Here's how the part is built. I have some questions about the finished solid (model axes, mm). Coordinates: 2 decimals unless noted, no trailing zeros. Loops run counter-clockwise (first coordinate to the right, second up) from the corner with the lowest first, then second, coordinate; pieces in that order, holes last. Notation, with made-up numbers: (81.5, 53.25) -> (126.5, 53.25) arc R31 ccw to (126.5, 83.25) -> close; hole circle Ø4 at (61, 71.25). An arc over 180 degrees is marked (long way). Answer as a JSON object with one key per item and string values. Group by question number.
1) I want a section at B-B (z = 2.25). Count the separate pieces of the cut face and the enclosed holes in it, then the cut area to 3 significant figures.
2) I need wall thicknesses on probe 1 along Y at (x, z) = (217, 1.25); probe 2 along X at (y, z) = (39, 1.25); probe 3 along Y at (x, z) = (42.5, 4.7). Which ranges of each line are inside material? Lowest first, please. Write a range as [from, to].
3) I want a section at A-A (y = 19). Write out the boundary of the cut face in (x, z).
4) I'm going to push flat-ended pins straight in: pin 1 (0.8 mm diameter, centred on x = 124, z = 3, fed in from +Y); pin 2 (2.5 mm diameter, centred on x = 99, z = 4, fed in from -Y); pin 3 (0.9 mm diameter, centred on x = 207.5, z = 3, fed in from -Y). Where does each tip first touch, or does it pass through?
Autodesk Inventor part; units mm, degrees
ref_plane "YZ Plane" through (0, 0, 0) normal (1, 0, 0) x (0, 1, 0)
ref_plane "XZ Plane" through (0, 0, 0) normal (0, 1, 0) x (-1, 0, 0)
ref_plane "XY Plane" through (0, 0, 0) normal (0, 0, 1) x (1, 0, 0)
sketch "Эскиз1" plane through (0, 0, 0) normal (0, 0, 1) x (1, 0, 0)
  line L0 (220, 84) -> (220, 0)
  line L1 (220, 0) -> (0, 0)
  line L2 (0, 0) -> (0, 84)
  line L3 (6, 0) -> (0, 0)
  line L4 (0, 76) -> (6, 76)
  line L5 (6, 76) -> (6, 8)
  line L6 (6, 8) -> (0, 8)
  line L7 (0, 8) -> (0, 76)
  ellipse E0 centre (95, 84) end of major axis (170, 84) minor radius 28.3094 (20, 84) -> (170, 84) ccw
  line L8 (0, 84) -> (20, 84)
  line L9 (170, 84) -> (220, 84)
  line L10 (220, 76) -> (214, 76)
  line L11 (214, 76) -> (214, 8)
  line L12 (214, 8) -> (220, 8)
  line L13 (220, 8) -> (220, 76)
  line L14 (0, 68) -> (6, 68)
  line L15 (6, 68) -> (6, 52)
  line L16 (6, 52) -> (0, 52)
  line L17 (0, 52) -> (0, 68)
  line L18 (0, 32) -> (6, 32)
  line L19 (6, 32) -> (6, 16)
  line L20 (6, 16) -> (0, 16)
  line L21 (0, 16) -> (0, 32)
  line L22 (214, 68) -> (220, 68)
  line L23 (214, 52) -> (220, 52)
  line L24 (214, 32) -> (220, 32)
  line L25 (214, 16) -> (220, 16)
  line L26 (0, 84) -> (-6, 84)
  line L27 (-6, 84) -> (-6, 0)
  line L28 (-6, 0) -> (0, 0)
  line L29 (0, 0) -> (0, 84)
  line L30 (220, 84) -> (226, 84)
  line L31 (226, 84) -> (226, 0)
  line L32 (226, 0) -> (220, 0)
  line L33 (220, 0) -> (220, 84)
  point P0 (217, 8)
  point P1 (220, 8)
  point P2 (3, 76)
  point P3 (3, 0)
  point P4 (217, 76)
  point P5 (3, 68)
  point P6 (0, 16)
  point P7 (0, 52)
  point P8 (217, 68)
  point P9 (217, 32)
  point P10 (217, 16)
  point P11 (217, 52)
  point P12 (220, 32)
  point P13 (220, 52)
  point P14 (220, 68)
  dimension "d1" = 75
  dimension "d0" = 220
  dimension "d2" = 125
  dimension "d3" = 84
  dimension "d4" = 150
  dimension "d5" = 84
  dimension "d6" = 6
  dimension "d7" = 8
  dimension "d10" = 6
  dimension "d11" = 8
  dimension "d12" = 8
  dimension "d13" = 8
  dimension "d14" = 84
  dimension "d35" = 8
  dimension "d36" = 8
  dimension "d37" = 16
  dimension "d38" = 16
  dimension "d39" = 8
  dimension "d40" = 8
  dimension "d41" = 16
  dimension "d42" = 16
  dimension "d96" = 6
  dimension "d97" = 6
extrude "Выдавливание1" add sketch "Эскиз1" along normal blind 6 contours L30 L31 L32 L0 | L0 L10 L11 L12 L1 L2 L6 L5 L4 L8 E0 L9 | L0 L23 L11 L22 | L2 L28 L27 L26 | L0 L25 L11 L24 | L14 L5 L16 L2 | L18 L5 L20 L2
sketch "Эскиз2" plane through (0, 0, 6) normal (0, 0, 1) x (1, 0, 0)
  line L0 (0, 0) -> (220, 0)
  line L1 (6, 0) -> (48, 0)
  line L2 (48, 0) -> (48, 8)
  line L3 (48, 8) -> (6, 8)
  line L4 (6, 8) -> (6, 0)
  line L5 (48, 0) -> (40, 0)
  line L6 (40, 0) -> (40, 42)
  line L7 (40, 42) -> (48, 42)
  line L8 (48, 42) -> (48, 0)
  line L9 (48, 42) -> (6, 42)
  line L10 (6, 42) -> (6, 34)
  line L11 (6, 34) -> (48, 34)
  line L12 (48, 34) -> (48, 42)
  line L13 (6, 42) -> (14, 42)
  line L14 (14, 42) -> (14, 0)
  line L15 (14, 0) -> (6, 0)
  line L16 (6, 0) -> (6, 42)
  line L17 (6, 16) -> (6, 8)
  circle A0 centre (11.5, 36.5) radius 1.5
  circle A1 centre (42.5, 36.5) radius 1.5
  circle A2 centre (42.5, 5.5) radius 1.5
  circle A3 centre (11.5, 5.5) radius 1.5
  circle A4 centre (184, 19) radius 7
  circle A5 centre (177, 25.9159) radius 1.5
  circle A6 centre (191, 26.0852) radius 1.5
  circle A7 centre (191, 12) radius 1.5
  circle A8 centre (177, 12) radius 1.5
  line L18 (177, 42.7055) -> (177, 0) construction
  line L19 (173.1146, 12) -> (210.5161, 12) construction
  line L20 (0, 0) -> (220, 0)
  line L21 (174.3072, 25.8833) -> (201.7049, 26.2146) construction
  line L22 (191, 29.1476) -> (191, 5.5) construction
  line L23 (214, 8) -> (214, 16)
  circle A9 centre (27, 21) radius 12.5
  point P0 (27, 0)
  point P1 (6, 76)
  point P2 (14, 34)
  point P3 (14, 8)
  point P4 (40, 8)
  point P5 (40, 34)
  dimension "d15" = 42
  dimension "d16" = 42
  dimension "d17" = 8
  dimension "d18" = 8
  dimension "d19" = 8
  dimension "d20" = 8
  dimension "d21" = 3
  dimension "d22" = 3
  dimension "d23" = 3
  dimension "d24" = 3
  dimension "d25" = 5.5
  dimension "d26" = 5.5
  dimension "d27" = 5.5
  dimension "d28" = 5.5
  dimension "d29" = 5.5
  dimension "d30" = 5.5
  dimension "d31" = 5.5
  dimension "d32" = 5.5
  dimension "d78" = 14
  dimension "d80" = 3
  dimension "d81" = 3
  dimension "d82" = 3
  dimension "d83" = 3
  dimension "d91" = 30
  dimension "d93" = 21
  dimension "d94" = 21
  dimension "d95" = 25
extrude "Выдавливание2" cut sketch "Эскиз2" against normal blind 6 contours A0 | A1 | A2 | A3 | A4 | A5 | A6 | A7 | A8 | A9
ref_plane "РабПлоскость1" through (110, 8, 0) normal (-1, 0, 0) x (0, 0, 1)
sketch "Эскиз5" plane through (0, 0, 0) normal (0, -1, 0) x (1, 0, 0)
  circle A0 centre (115, 3) radius 1.5
  circle A1 centre (105, 3) radius 1.5
  line L0 (110, -1.2) -> (110, 7.2)
  line L1 (0, 0) -> (220, 0)
  dimension "d70" = 5
  dimension "d71" = 5
  dimension "d72" = 3
  dimension "d73" = 3
  dimension "d74" = 3
  dimension "d75" = 3
extrude "Выдавливание3" [suppressed]
fillet "Сопряжение1" radius 5 2 edges at (170, 84, 3) (20, 84, 3)
sketch "Эскиз6" plane through (0, 0, 6) normal (0, 0, 1) x (1, 0, 0)
  line L0 (-6, 0) -> (226, 0)
  line L1 (100, 0) -> (97, 0)
  line L2 (97, 0) -> (97, 10)
  line L3 (97, 10) -> (100, 10)
  line L4 (100, 10) -> (100, 0)
  line L5 (123, 0) -> (120, 0)
  line L6 (120, 0) -> (120, 10)
  line L7 (120, 10) -> (123, 10)
  line L8 (123, 10) -> (123, 0)
  line L9 (124.5, 4.2) -> (118.5, 4.2)
  line L10 (118.5, 4.2) -> (118.5, 1.8)
  line L11 (118.5, 1.8) -> (124.5, 1.8)
  line L12 (124.5, 1.8) -> (124.5, 4.2)
  line L13 (95.5, 4.2) -> (101.5, 4.2)
  line L14 (101.5, 4.2) -> (101.5, 1.8)
  line L15 (101.5, 1.8) -> (95.5, 1.8)
  line L16 (95.5, 1.8) -> (95.5, 4.2)
  line L17 (110, -16.8) -> (110, 100.8)
  point P0 (0, 0)
  point P1 (120, 1.8)
  point P2 (120, 0)
  point P3 (123, 1.8)
  point P4 (123, 4.2)
  point P5 (120, 4.2)
  point P6 (97, 1.8)
  point P7 (97, 0)
  point P8 (100, 1.8)
  point P9 (100, 4.2)
  point P10 (97, 4.2)
  dimension "d98" = 10
  dimension "d99" = 10
  dimension "d100" = 13
  dimension "d101" = 3
  dimension "d102" = 3
  dimension "d103" = 10
  dimension "d104" = 6
  dimension "d105" = 8.5
  dimension "d106" = 2.4
  dimension "d107" = 1.8
  dimension "d108" = 2.4
  dimension "d109" = 6
  dimension "d110" = 8.5
extrude "Выдавливание4" cut sketch "Эскиз6" against normal blind 6
sketch "Эскиз7" plane through (0, 0, 6) normal (0, 0, 1) x (1, 0, 0)
  circle A0 centre (3, 60) radius 1.5
  circle A1 centre (3, 24) radius 1.5
  line L0 (6, 68) -> (0, 68)
  line L1 (6, 76) -> (6, 68) construction
  line L2 (0, 52) -> (6, 52) construction
  line L3 (6, 68) -> (6, 52) construction
  line L4 (6, 32) -> (0, 32) construction
  point P0 (0, 0)
  point P1 (3, 68)
  point P2 (3, 32)
  dimension "d113" = 3
  dimension "d114" = 3
  dimension "d115" = 8
  dimension "d116" = 3
  dimension "d118" = 8
  dimension "d119" = 3
extrude "Выдавливание5" cut sketch "Эскиз7" against normal blind 6
mirror "Зеркальное отражение2" about plane through (110, 8, 0) normal (-1, 0, 0) of "Выдавливание5"
sketch "Эскиз8" plane through (0, 0, 6) normal (0, 0, 1) x (1, 0, 0)
  circle A0 centre (217, 24) radius 1.5
  circle A1 centre (217, 60) radius 1.5
  circle A2 centre (3, 24) radius 1.5
  circle A3 centre (3, 60) radius 1.5
  line L0 (0, 8) -> (0, 16)
  line L1 (0, 16) -> (6, 16)
  line L2 (6, 16) -> (6, 8)
  line L3 (6, 8) -> (0, 8)
  line L4 (0, 32) -> (0, 52)
  line L5 (0, 52) -> (6, 52)
  line L6 (6, 52) -> (6, 32)
  line L7 (6, 32) -> (0, 32)
  line L8 (0, 68) -> (0, 76)
  line L9 (0, 76) -> (6, 76)
  line L10 (6, 76) -> (6, 68)
  line L11 (6, 68) -> (0, 68)
  line L12 (220, 76) -> (220, 68)
  line L13 (220, 68) -> (214, 68)
  line L14 (214, 68) -> (214, 76)
  line L15 (214, 76) -> (220, 76)
  line L16 (220, 52) -> (220, 32)
  line L17 (220, 32) -> (214, 32)
  line L18 (214, 32) -> (214, 52)
  line L19 (214, 52) -> (220, 52)
  line L20 (220, 16) -> (220, 8)
  line L21 (220, 8) -> (214, 8)
  line L22 (214, 8) -> (214, 16)
  line L23 (214, 16) -> (220, 16)
  circle A4 centre (27, 21) radius 12.5
  circle A5 centre (177, 12) radius 1.5
  circle A6 centre (42.5, 5.5) radius 1.5
  circle A7 centre (42.5, 36.5) radius 1.5
  circle A8 centre (177, 25.9159) radius 1.5
  circle A9 centre (184, 19) radius 7
  circle A10 centre (191, 12) radius 1.5
  circle A11 centre (11.5, 5.5) radius 1.5
  circle A12 centre (11.5, 36.5) radius 1.5
  circle A13 centre (191, 26.0852) radius 1.5
  line L24 (120, 0) -> (120, 1.8)
  line L25 (120, 1.8) -> (118.5, 1.8)
  line L26 (118.5, 1.8) -> (118.5, 4.2)
  line L27 (118.5, 4.2) -> (120, 4.2)
  line L28 (120, 4.2) -> (120, 10)
  line L29 (120, 10) -> (123, 10)
  line L30 (123, 10) -> (123, 4.2)
  line L31 (123, 4.2) -> (124.5, 4.2)
  line L32 (124.5, 4.2) -> (124.5, 1.8)
  line L33 (124.5, 1.8) -> (123, 1.8)
  line L34 (123, 1.8) -> (123, 0)
  line L35 (123, 0) -> (226, 0)
  line L36 (226, 0) -> (226, 84)
  line L37 (226, 84) -> (174.1947, 84)
  arc A14 (174.1947, 84) -> (169.4402, 80.5476) centre (174.1947, 79) ccw
  ellipse E0 centre (95, 84) end of major axis (20, 84) minor radius 28.3094 (20.5598, 80.5476) -> (169.4402, 80.5476) ccw
  arc A15 (20.5598, 80.5476) -> (15.8053, 84) centre (15.8053, 79) ccw
  line L38 (15.8053, 84) -> (-6, 84)
  line L39 (-6, 84) -> (-6, 0)
  line L40 (-6, 0) -> (97, 0)
  line L41 (97, 0) -> (97, 1.8)
  line L42 (97, 1.8) -> (95.5, 1.8)
  line L43 (95.5, 1.8) -> (95.5, 4.2)
  line L44 (95.5, 4.2) -> (97, 4.2)
  line L45 (97, 4.2) -> (97, 10)
  line L46 (97, 10) -> (100, 10)
  line L47 (100, 10) -> (100, 4.2)
  line L48 (100, 4.2) -> (101.5, 4.2)
  line L49 (101.5, 4.2) -> (101.5, 1.8)
  line L50 (101.5, 1.8) -> (100, 1.8)
  line L51 (100, 1.8) -> (100, 0)
  line L52 (100, 0) -> (120, 0)
  line L53 (214, 58.5) -> (220, 58.5)
  line L54 (220, 58.5) -> (220, 52)
  line L55 (214, 52) -> (220, 52)
  line L56 (214, 32) -> (214, 52)
  line L57 (220, 32) -> (214, 32)
  line L58 (220, 32) -> (220, 25.5)
  line L59 (220, 25.5) -> (214, 25.5)
  line L60 (214, 25.5) -> (214, 32)
  line L61 (214, 52) -> (214, 58.5)
  line L62 (220, 52) -> (220, 32)
  line L63 (220, 61.5) -> (214, 61.5)
  line L64 (214, 61.5) -> (214, 68)
  line L65 (214, 68) -> (214, 76)
  line L66 (214, 76) -> (214, 84)
  line L67 (214, 84) -> (220, 84)
  line L68 (220, 84) -> (220, 76)
  line L69 (220, 76) -> (220, 68)
  line L70 (220, 68) -> (220, 61.5)
  line L71 (220, 68) -> (214, 68)
  line L72 (214, 76) -> (220, 76)
  line L73 (214, -6) -> (214, 8)
  line L74 (214, 8) -> (214, 16)
  line L75 (214, 16) -> (214, 22.5)
  line L76 (214, 22.5) -> (220, 22.5)
  line L77 (220, 22.5) -> (220, 16)
  line L78 (220, 16) -> (220, 8)
  line L79 (220, 8) -> (220, -6)
  line L80 (220, -6) -> (214, -6)
  line L81 (220, 8) -> (214, 8)
  line L82 (214, 16) -> (220, 16)
  line L83 (209, 0) -> (206, 0)
  line L84 (206, 0) -> (206, 10)
  line L85 (206, 10) -> (209, 10)
  line L86 (209, 10) -> (209, 0)
  line L87 (204.5, 4.4) -> (210.5, 4.4)
  line L88 (210.5, 4.4) -> (210.5, 2)
  line L89 (210.5, 2) -> (204.5, 2)
  line L90 (204.5, 2) -> (204.5, 4.4)
  point P0 (0, 0)
  point P1 (204.5, 3.2)
  point P2 (207.5, 0)
  point P3 (206, 4.4)
  point P4 (206, 2)
  point P5 (209, 2)
  point P6 (209, 4.4)
  dimension "d122" = 5
  dimension "d123" = 3
  dimension "d124" = 2.4
  dimension "d125" = 6
  dimension "d126" = 1.5
  dimension "d127" = 2
  dimension "d128" = 10
extrude "Выдавливание6" cut sketch "Эскиз8" against normal through all contours L35 L84 L89 L86 | L89 L84 L87 L86 | L86 L87 L88 L89 | L89 L90 L87 L84 | L87 L84 L85 L86
equation "\"d36\" = d35"
equation "\"d22\" = d21"
equation "\"d23\" = d21"
equation "\"d24\" = d21"
properties part number "боковая стенка"
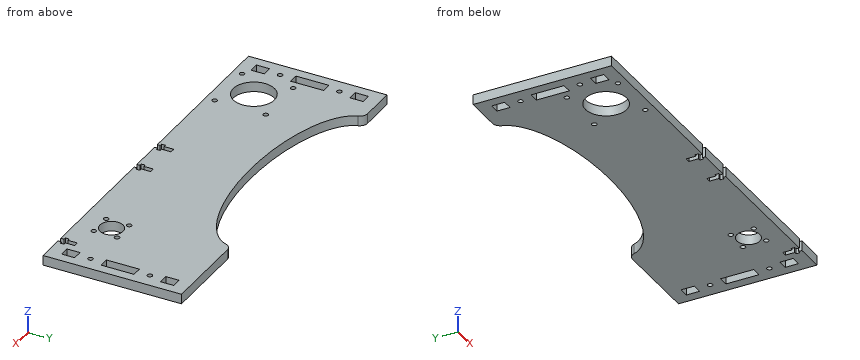
Determined:
{
 "1": {"separate pieces": "1", "enclosed holes": "20", "area": "14,900 mm^2"},
 "2": {"probe 1": "[0, 8], [16, 22.5], [25.5, 32], [52, 58.5], [61.5, 68], [76, 84]", "probe 2": "[-6, 0], [6, 214], [220, 226]", "probe 3": "[0, 4], [7, 35], [38, 63.78]"},
 "3": {"outline": "(-6, 0) -> (14.66, 0) -> (14.66, 6) -> (-6, 6) -> close; (39.34, 0) -> (177, 0) -> (177, 6) -> (39.34, 6) -> close; (191, 0) -> (226, 0) -> (226, 6) -> (191, 6) -> close"},
 "4": {"pin 1": "y = 57.96", "pin 2": "y = 0", "pin 3": "y = 10"}
}
